Part model, mm, in its own coordinate system. Give positions to 0.01 mm unless a question says otherwise; leave off trailing zeros. Order: outer loops, then holes, each group sorted by start corner. A loop starts at its lowest first (then second) coordinate and runs counter-clockwise, first axis right, second up. Notation, with made-up numbers: (-16.75, 46.5) -> (30.25, 46.5) arc R31 cw to (30.25, 72.5) -> close; hole circle Ø3 at (69, -6.75). An arc over 180 degrees is marked (long way). Write item = value, one per line. Start each with the question number.
(1) Saw through at B-B, the plane z = 29. List the corners of the cut face in (x, y), then the cut area to 3 significant figures.
(2) Probe line 1 along Y through (x, z) = (3, 46); line 2 along Y through (x, z) = (0.25, 46.5); line 3 along X through (y, z) = (31.5, 37.5). List the from-to ranges inside material, lowest first. Write a range as from..to.
(3) Saw through at D-D, the plane z = 62. List the corners of the cut face in (x, y).
(4) Flat gauge pins, fed straight in: pin 1 (0.6 mm diameter, centred on x = -1, z = 59, fed in from -Y); pin 2 (2 mm diameter, centred on x = 2.5, z = 57, fed in from +Y); pin 3 (1.6 mm diameter, centred on x = -0.5, y = 10.5, fed in from +Z); pin 4 (4.5 mm diameter, centred on y = 10, z = 28.14, fed in from -X). Where does each tip first touch, or does it go through?
(5) Saw through at C-C, the plane x = 2. List the corners of the cut face in (y, z) (3 decimals), then the cut area to 3 significant figures.
(6) Saw through at A-A, the plane y = 10. List the corners of the cut face in (x, z), then the cut area to 3 significant figures.
from build123d import *

# Parameters (mm, degrees)
BOSS_EXTRUDE1_DEPTH      = 4
SKETCH2_R                = 2.375
CUT_EXTRUDE1_DEPTH       = 5
LPATTERN1_COUNT          = 3
LPATTERN1_PITCH          = 20
SKETCH2_4_R              = 2.375
CUT_EXTRUDE2_DEPTH       = 5
LPATTERN2_COUNT          = 2
LPATTERN2_PITCH          = 20
FILLET1_R                = 3
CHANFRO1_SIZE            = 1
RESSALTO_EXTRUS_O1_START = -4
ESBO_O1_W                = 10
ESBO_O1_H                = 6
RESSALTO_EXTRUS_O1_DEPTH = 2


with BuildPart() as part:
    # Sketch1 → Boss-Extrude1 (new body)
    with BuildSketch(Plane(origin=(0, 0, 0), x_dir=(0, 0, -1), z_dir=(1, 0, 0))):
        Polygon((-78.140120378, 0), (-18.140120378, 0), (-18.140120378, 18.140120378), (-58.68306962, 58.68306962), (-71.510071751, 45.856067489), (-78.140120378, 18.140120378), align=None)
    extrude(amount=BOSS_EXTRUDE1_DEPTH)

    # Sketch2 → Cut-Extrude1 (cut, through all)
    with BuildSketch(Plane(origin=(4, 0, 0), x_dir=(0, 0, -1), z_dir=(1, 0, 0))):
        with Locations((-28.140120378, 10)):
            Circle(SKETCH2_R)
    cut_extrude1 = extrude(amount=-CUT_EXTRUDE1_DEPTH, mode=Mode.SUBTRACT)

    # LPattern1: Cut-Extrude1 ×3
    with Locations(*[(0, 0, i * LPATTERN1_PITCH) for i in range(1, LPATTERN1_COUNT)]):
        add(cut_extrude1, mode=Mode.SUBTRACT)

    # Sketch2_4 → Cut-Extrude2 (cut, through all)
    with BuildSketch(Plane(origin=(4, 0, 0), x_dir=(0, 0, -1), z_dir=(1, 0, 0))):
        with Locations((-58.68306962, 44.540933996)):
            Circle(SKETCH2_4_R)
    cut_extrude2 = extrude(amount=-CUT_EXTRUDE2_DEPTH, mode=Mode.SUBTRACT)

    # LPattern2: Cut-Extrude2 ×2
    with Locations(*[Vector(0, -0.707106781, -0.707106781) * (i * LPATTERN2_PITCH) for i in range(1, LPATTERN2_COUNT)]):
        add(cut_extrude2, mode=Mode.SUBTRACT)

    # Fillet1
    fillet1_edges = [part.edges().sort_by_distance(p)[0] for p in [
        (2, 18.140120378, 78.140120378),
        (2, 45.856067489, 71.510071751),
        (2, 58.68306962, 58.68306962),
        (2, 18.140120378, 18.140120378),
        (2, 0, 18.140120378),
        (2, 0, 78.140120378),
    ]]
    fillet(fillet1_edges, radius=FILLET1_R)

    # Chanfro1
    chanfro1_edges = [part.edges().sort_by_distance(p)[0] for p in [
        (0, 0, 48.140120378),
        (4, 0, 48.140120378),
        (0, 10.393145239, 78.140120378),
        (0, 31.75807492, 74.882512025),
        (0, 51.508513622, 65.857625619),
        (0, 37.790274655, 37.790274655),
        (0, 9.948739845, 18.140120378),
        (0, 57.440428933, 58.68306962),
        (0, 18.045529988, 18.36848178),
        (0, 0.878679656, 19.018800034),
        (0, 45.798751214, 71.407627967),
        (0, 18.137684762, 78.119469645),
        (0, 0.878679656, 77.261440721),
        (4, 10.393145239, 78.140120378),
        (4, 9.948739845, 18.140120378),
        (4, 37.790274655, 37.790274655),
        (4, 51.508513622, 65.857625619),
        (4, 31.75807492, 74.882512025),
        (4, 57.440428933, 58.68306962),
        (4, 18.045529988, 18.36848178),
        (4, 0.878679656, 19.018800034),
        (4, 45.798751214, 71.407627967),
        (4, 18.137684762, 78.119469645),
        (4, 0.878679656, 77.261440721),
    ]]
    chamfer(chanfro1_edges, length=CHANFRO1_SIZE)

    # Esbo_o1 → Ressalto-extrus_o1 (add)
    with BuildSketch(Plane(origin=(4, 0, 0), x_dir=(0, 0, -1), z_dir=(1, 0, 0)).offset(RESSALTO_EXTRUS_O1_START)):
        Polygon((-57.21666665, 39.183379746), (-50.59244791, 31.692069708), (-46.097661887, 35.666600952), (-52.721880627, 43.15791099), align=None)
        with Locations((-58.140120378, 10)):
            Rectangle(ESBO_O1_W, ESBO_O1_H)
        with Locations((-38.140120378, 10)):
            Rectangle(ESBO_O1_W, ESBO_O1_H)
    extrude(amount=-RESSALTO_EXTRUS_O1_DEPTH)


solid = part.part
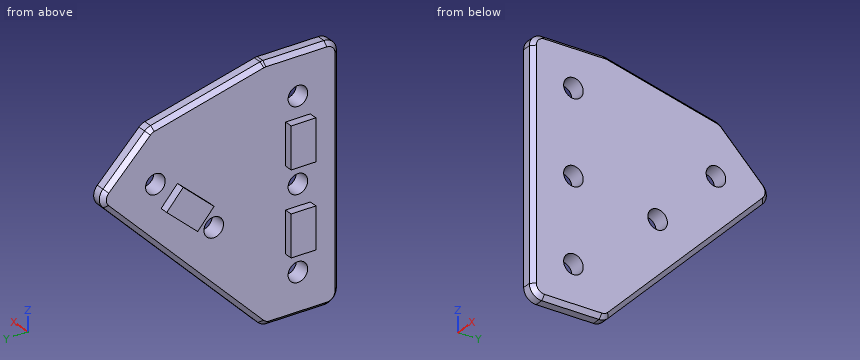
Results list:
q1.outline = (0, 1) -> (1, 0) -> (3, 0) -> (4, 1) -> (4, 7.79) -> (0, 7.79) -> close; (0, 12.21) -> (4, 12.21) -> (4, 27.59) -> (3, 29) -> (1, 29) -> (0, 27.59) -> close
q1.area = 95.9 mm^2
q2.line_1 = 0..8.97, 11.03..28.52, 32.27..46
q2.line_2 = 0.75..8.28, 11.72..29.06, 31.74..45.44
q2.line_3 = 0..4
q3.outline = (-2, 7) -> (0, 7) -> (0, 1) -> (1, 0) -> (3, 0) -> (4, 1) -> (4, 53.95) -> (3, 55.37) -> (1, 55.37) -> (0, 53.95) -> (0, 13) -> (-2, 13) -> close
q4.pin_1 = 7
q4.pin_2 = 57.36
q4.pin_3 = 77.44
q4.pin_4 = through
q5.outline = (0, 21.14) arc R3 ccw to (3, 18.14) -> (16.897, 18.14) arc R3 ccw to (19.019, 19.019) -> (56.562, 56.562) arc R3 ccw to (56.562, 60.804) -> (46.455, 70.911) arc R3 ccw to (45.032, 71.707) -> (18.484, 78.058) arc R3 ccw to (17.786, 78.14) -> (3, 78.14) arc R3 ccw to (0, 75.14) -> close; hole circle Ø4.75 at (10, 28.14); hole circle Ø4.75 at (10, 48.14); hole circle Ø4.75 at (10, 68.14); hole circle Ø4.75 at (30.399, 44.541); hole circle Ø4.75 at (44.541, 58.683)
q5.area = 2,350 mm^2
q6.outline = (-2, 33.14) -> (0, 33.14) -> (0, 30.52) -> (4, 30.52) -> (4, 45.77) -> (0, 45.77) -> (0, 43.14) -> (-2, 43.14) -> close; (-2, 53.14) -> (0, 53.14) -> (0, 50.52) -> (4, 50.52) -> (4, 65.77) -> (0, 65.77) -> (0, 63.14) -> (-2, 63.14) -> close; (0, 19.14) -> (1, 18.14) -> (3, 18.14) -> (4, 19.14) -> (4, 25.77) -> (0, 25.77) -> close; (0, 70.52) -> (4, 70.52) -> (4, 77.14) -> (3, 78.14) -> (1, 78.14) -> (0, 77.14) -> close
q6.area = 221 mm^2
